Source: CAD feature listing. Evaluate the final solid. Frame: model axes, mm. A direction names the side the tool comes from. Round coordinates to 2 decimals unless told otherwise and drop trailing zeros. Loops run counter-clockwise (first coordinate to the right, second up) from the corner with the lowest first, then second, coordinate; pieces in that order, holes last. Notation, with made-up numbers: (46, -16) - (62, -16) arc R21 cw to (62, 15) - close; hole circle Ø4 at (45, 4.5). An arc over 180 degrees is marked (long way). One line per question, with ' | ' between items.
from build123d import *

# Parameters (mm, degrees)
SKETCH1_W           = 130
SKETCH1_H           = 75
BOSS_EXTRUDE1_DEPTH = 6
SKETCH2_R           = 8
CUT_EXTRUDE1_DEPTH  = 151.203195705
SKETCH3_W           = 26
SKETCH3_H           = 4
CUT_EXTRUDE2_DEPTH  = 151.203195705
CUT_EXTRUDE3_DEPTH  = 151.203195705


with BuildPart() as part:
    # Sketch1 → Boss-Extrude1 (new body)
    with BuildSketch(Plane(origin=(0, 0, 0), x_dir=(1, 0, 0), z_dir=(0, 1, 0))):
        with Locations((65, 37.5)):
            Rectangle(SKETCH1_W, SKETCH1_H)
    extrude(amount=BOSS_EXTRUDE1_DEPTH)

    # Sketch2 → Cut-Extrude1 (cut, through all)
    with BuildSketch(Plane(origin=(0, 6, 0), x_dir=(1, 0, 0), z_dir=(0, 1, 0))):
        with Locations(Location((52.25, 18.25, 0), (0, 0, 270))):
            Circle(SKETCH2_R)
        with Locations(Location((77.75, 18.25, 0), (0, 0, 270))):
            Circle(SKETCH2_R)
    extrude(amount=-CUT_EXTRUDE1_DEPTH, mode=Mode.SUBTRACT)

    # Sketch3 → Cut-Extrude2 (cut, through all)
    with BuildSketch(Plane(origin=(0, 6, 0), x_dir=(1, 0, 0), z_dir=(0, 1, 0))):
        Polygon((0, 75), (0, 50), (6, 50), (6, 69), (43, 69), (43, 75), align=None)
        Polygon((87, 75), (87, 69), (124, 69), (124, 50), (130, 50), (130, 75), align=None)
        with Locations((13, 43)):
            Rectangle(SKETCH3_W, SKETCH3_H)
        Polygon((6, 25), (0, 25), (0, 0), (43, 0), (43, 6), (6, 6), align=None)
        with Locations((65, 43)):
            Rectangle(SKETCH3_W, SKETCH3_H)
        with Locations((117, 43)):
            Rectangle(SKETCH3_W, SKETCH3_H)
        Polygon((130, 25), (124, 25), (124, 6), (87, 6), (87, 0), (130, 0), align=None)
    extrude(amount=-CUT_EXTRUDE2_DEPTH, mode=Mode.SUBTRACT)

    # Sketch4 → Cut-Extrude3 (cut, through all)
    with BuildSketch(Plane(origin=(0, 6, 0), x_dir=(1, 0, 0), z_dir=(0, 1, 0))):
        with BuildLine():
            Line((102.5, 22.783882181), (102.5, 17.216117819))
            ThreePointArc((102.5, 17.216117819), (110, 12), (117.5, 17.216117819))
            Line((117.5, 17.216117819), (117.5, 22.783882181))
            ThreePointArc((117.5, 22.783882181), (110, 28), (102.5, 22.783882181))
        make_face()
    extrude(amount=-CUT_EXTRUDE3_DEPTH, mode=Mode.SUBTRACT)


solid = part.part
1. Material intervals for probe 1 along X at (y, z) = (3.3, -18.25); probe 2 along X at (y, z) = (1.5, -44); probe 3 along Z at (x, y) = (16.5, 4.55), sorted ascending.
Worked out:
probe 1: x = 6 to 44.25, 60.25 to 69.75, 85.75 to 102.5, 117.5 to 124 | probe 2: x = 26 to 52, 78 to 104 | probe 3: z = -69 to -45, -41 to -6
2. Section query C-C, the plane x = 73.5. Return loops of the section in (y, z).
Worked out:
outline: (0, -75) - (6, -75) - (6, -45) - (0, -45) - close; (0, -41) - (6, -41) - (6, -25.03) - (0, -25.03) - close; (0, -11.47) - (6, -11.47) - (6, 0) - (0, 0) - close
3. Access query for faces 4 (the flat face through (124, 3, -60)), 5 (the flat face through (104, 3, -43)), 6 (the flat face through (117.5, 3, -20)), 7 (the flat face through (25, 3, -6)). Directions: +Z, -Z, +X, -X, +Y, -Y. A direction counts if a zero-diameter tool reaches every point of the face in a straight line with its end or side. Return the directions, or none.
Worked out:
face 4: -Z, +X, +Y, -Y | face 5: +X, +Y, -Y | face 6: +Y, -Y | face 7: +Z, -X, +Y, -Y
4. Section query D-D, the plane z = -18.5. Return loops of the section in (x, y), plus the area to 3 significant figures.
Worked out:
outline: (6, 0) - (44.25, 0) - (44.25, 6) - (6, 6) - close; (60.25, 0) - (69.75, 0) - (69.75, 6) - (60.25, 6) - close; (85.75, 0) - (102.5, 0) - (102.5, 6) - (85.75, 6) - close; (117.5, 0) - (124, 0) - (124, 6) - (117.5, 6) - close | area: 426 mm2
5. Section query B-B, the plane z = -43.5. Return loops of the section in (x, y), plus the area to 3 significant figures.
Worked out:
outline: (26, 0) - (52, 0) - (52, 6) - (26, 6) - close; (78, 0) - (104, 0) - (104, 6) - (78, 6) - close | area: 312 mm2
6. Contact query for flat-ended pins moving along their axis: P1, Ø1.8, axis at x = 3.5, y = 4, coming from the -Z side; P2, Ø2, axis at y = 3.5, z = -58, coming from the -X side; P3, Ø1.8, axis at x = 111.5, y = 2, coming from the -Z side. Output: stop coordinate, or through.
Worked out:
P1: stops at z = -50 | P2: stops at x = 6 | P3: stops at z = -69
7. Section query A-A, the plane x = 21.5. Return loops of the section in (y, z), plus the area to 3 significant figures.
Worked out:
outline: (0, -69) - (6, -69) - (6, -45) - (0, -45) - close; (0, -41) - (6, -41) - (6, -6) - (0, -6) - close | area: 354 mm2
8. Mould query, pull axis X, two halves, no side actions, for faces 1 (the flat face through (130, 3, -47)), 2 (the flat face through (78, 3, -43)), 3 (the flat face through (6, 3, -15)). Classes: released by +X, released by -X, zero draft, split by the parting line, or undercut.
Worked out:
face 1: released by +X | face 2: undercut | face 3: released by -X
